Build history of the part. All positions in model axes, mm. Face numbers are marked on the shaded views. Round coordinates to 2 decimals unless told otherwise and drop trailing zeros. Order: outer loops, then holes, each group sorted by start corner. A loop starts at its lowest first (then second) coordinate and runs counter-clockwise, first axis right, second up. Notation, with made-up numbers: M 25.5,-10.75 L 78.5,-10.75 A32 cw 78.5,22.25 Z; hole C 5,45 d8. An arc over 180 degrees is marked long. One line per item, written item: value. Start each with the question number.
Item 1: Two-plate mould, pull along X, no slides. Class the marked faces 1, 2 and 3: +X half, -X half, draft (parallel to the pull), parting line (faces both ways), or undercut.
Item 2: Probe L1, parallel to Y at x = 0, z = 0.65; L2, parallel to X at y = 0, z = 8.75; L3, parallel to Y at x = 0, z = 6.25. List the from-to ranges inside material, lowest first.
Item 3: Band-saw the part on C-C, the plane y = 4.5. Write the cut outline in (x, z), then the cut area to 3 significant figures.
Item 4: Pin check, flat tips, straight feed: pin 1 (4 mm diameter, centred on x = 15, y = -23.5, fed in from +Z); pin 2 (1 mm diameter, centred on x = 11, z = 8.5, fed in from +Y); pin 3 (0.6 mm diameter, centred on y = -32.5, z = 1.5, fed in from -X). Stop position of each tip, or through.
Item 5: Band-saw the part on D-D, the plane x = 29.5. Write the cut outline in (y, z), then the cut area to 3 significant figures.
Item 6: Band-saw the part on A-A, the plane x = 0. Write the cut outline in (y, z), then the cut area to 3 significant figures.
Item 7: Band-saw the part on B-B, the plane y = 15. Write the cut outline in (x, z), then the cut area to 3 significant figures.
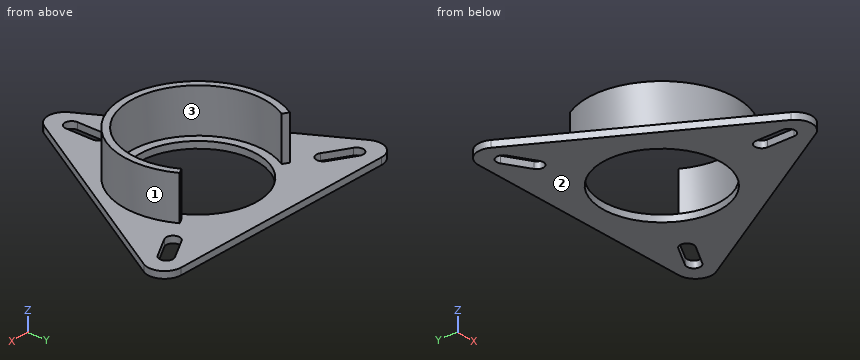
```python
from build123d import *

# Parameters (mm, degrees)
F0_R     = 17.5
F1_DEPTH = 2
F2_DEPTH = 15


with BuildPart() as f1:
    # F0 (on Top) → F1 (new body)
    with BuildSketch(Plane.XY):
        with BuildLine():
            Line((34.641016, 25), (-34.641016, 25))
            ThreePointArc((-34.641016, 25), (-38.971143, 22.5), (-38.971143, 17.5))
            Line((-38.971143, 17.5), (-4.330127, -42.5))
            ThreePointArc((-4.330127, -42.5), (0, -45), (4.330127, -42.5))
            Line((4.330127, -42.5), (38.971143, 17.5))
            ThreePointArc((38.971143, 17.5), (38.971143, 22.5), (34.641016, 25))
        make_face()
        with BuildLine():
            ThreePointArc((2, -38), (0, -40), (-2, -38))
            Line((-2, -38), (-2, -30))
            ThreePointArc((-2, -30), (0, -28), (2, -30))
            Line((2, -30), (2, -38))
        make_face(mode=Mode.SUBTRACT)
        with BuildLine():
            ThreePointArc((-33.908965, 17.267949), (-34.641016, 20), (-31.908965, 20.732051))
            Line((-31.908965, 20.732051), (-24.980762, 16.732051))
            ThreePointArc((-24.980762, 16.732051), (-24.248711, 14), (-26.980762, 13.267949))
            Line((-26.980762, 13.267949), (-33.908965, 17.267949))
        make_face(mode=Mode.SUBTRACT)
        with BuildLine():
            Line((-19.052559, 11), (-17.320508, 10))
            ThreePointArc((-17.320508, 10), (0, -20), (17.320508, 10))
            Line((17.320508, 10), (19.052559, 11))
            ThreePointArc((19.052559, 11), (0, -22), (-19.052559, 11))
        make_face(mode=Mode.SUBTRACT)
        Circle(F0_R, mode=Mode.SUBTRACT)
        with BuildLine():
            ThreePointArc((31.908965, 20.732051), (34.641016, 20), (33.908965, 17.267949))
            Line((33.908965, 17.267949), (26.980762, 13.267949))
            ThreePointArc((26.980762, 13.267949), (24.248711, 14), (24.980762, 16.732051))
            Line((24.980762, 16.732051), (31.908965, 20.732051))
        make_face(mode=Mode.SUBTRACT)
    extrude(amount=F1_DEPTH)

    # F0 (on Top) → F2 (join)
    with BuildSketch(Plane.XY):
        with BuildLine():
            ThreePointArc((17.320508, 10), (0, -20), (-17.320508, 10))
            Line((-17.320508, 10), (-19.052559, 11))
            ThreePointArc((-19.052559, 11), (0, -22), (19.052559, 11))
            Line((19.052559, 11), (17.320508, 10))
        make_face()
    extrude(amount=F2_DEPTH)


solid = f1.part
```
Output:
1. face 1: parting line
1. face 2: draft
1. face 3: undercut
2. L1: y = -45 to -40, -28 to -17.5, 17.5 to 25
2. L2: x = -22 to -20, 20 to 22
2. L3: y = -22 to -20
3. outline: M -31.47,0 L -16.91,0 L -16.91,2 L -19.49,2 L -19.49,15 L -21.53,15 L -21.53,2 L -31.47,2 Z; M 16.91,0 L 31.47,0 L 31.47,2 L 21.53,2 L 21.53,15 L 19.49,15 L 19.49,2 L 16.91,2 Z
3. area: 111 mm²
4. pin 1: stops at z = 2
4. pin 2: stops at y = -16.36
4. pin 3: stops at x = -10.28
5. outline: M 1.1,0 L 14.72,0 L 14.72,2 L 1.1,2 Z; M 19.34,0 L 25,0 L 25,2 L 19.34,2 Z
5. area: 38.6 mm²
6. outline: M -45,0 L -40,0 L -40,2 L -45,2 Z; M -28,0 L -17.5,0 L -17.5,2 L -20,2 L -20,15 L -22,15 L -22,2 L -28,2 Z; M 17.5,0 L 25,0 L 25,2 L 17.5,2 Z
6. area: 72.0 mm²
7. outline: M -37.53,0 L -29.98,0 L -29.98,2 L -37.53,2 Z; M -23.98,0 L -9.01,0 L -9.01,2 L -23.98,2 Z; M 9.01,0 L 23.98,0 L 23.98,2 L 9.01,2 Z; M 29.98,0 L 37.53,0 L 37.53,2 L 29.98,2 Z
7. area: 90.1 mm²
